Model file for the job. Use its own axes, mm. Round coordinates to 2 decimals unless told otherwise and drop trailing zeros. Loops run counter-clockwise (first coordinate to the right, second up) from the corner with the lowest first, then second, coordinate; pieces in that order, holes last. Notation, with made-up numbers: (-29.5, -10.75) -> (-1.5, -10.75) arc R9 cw to (-1.5, 5.25) -> close; hole circle Ø3 at (88.5, 75). An arc over 180 degrees is marked (long way). Use a Markdown table: item, result.
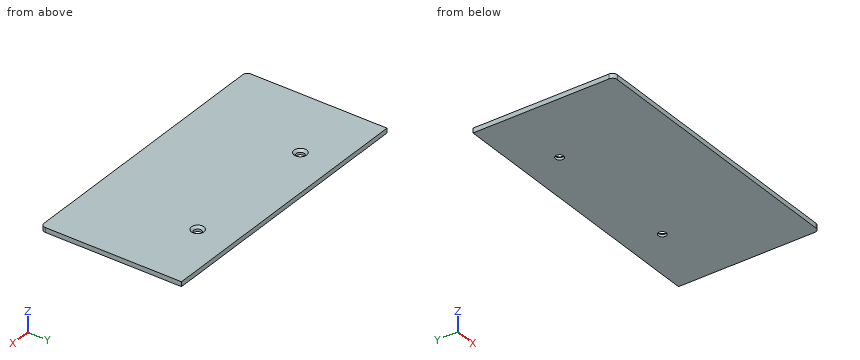
from build123d import *

# Parameters (mm, degrees)
SCHIZZO1_W                   = 120
SCHIZZO1_H                   = 60
SCHIZZO1_R                   = 1.7
ESTRUSIONE_ESTRUSIONE2_DEPTH = 2
RACCORDO1_R                  = 2
RACCORDO2_R                  = 2
SMUSSO1_SIZE                 = 1
SMUSSO2_SIZE                 = 1


with BuildPart() as part:
    # Schizzo1 → Estrusione-Estrusione2 (new body)
    with BuildSketch(Plane.XY):
        with Locations((60, 30)):
            Rectangle(SCHIZZO1_W, SCHIZZO1_H)
        with Locations((90, 45)):
            Circle(SCHIZZO1_R, mode=Mode.SUBTRACT)
        with Locations(Location((30, 45, 0), (0, 0, 180))):
            Circle(SCHIZZO1_R, mode=Mode.SUBTRACT)
    extrude(amount=-ESTRUSIONE_ESTRUSIONE2_DEPTH)

    # Raccordo1
    raccordo1_edges = [part.edges().sort_by_distance(p)[0] for p in [
        (0, 0, -1),
    ]]
    fillet(raccordo1_edges, radius=RACCORDO1_R)

    # Raccordo2
    raccordo2_edges = [part.edges().sort_by_distance(p)[0] for p in [
        (120, 0, -1),
    ]]
    fillet(raccordo2_edges, radius=RACCORDO2_R)

    # Smusso1
    smusso1_edges = [part.edges().sort_by_distance(p)[0] for p in [
        (31.7, 45, 0),
    ]]
    chamfer(smusso1_edges, length=SMUSSO1_SIZE)

    # Smusso2
    smusso2_edges = [part.edges().sort_by_distance(p)[0] for p in [
        (88.3, 45, 0),
    ]]
    chamfer(smusso2_edges, length=SMUSSO2_SIZE)


solid = part.part
Q1. Drill centre lines: L1, parallel to Y at x = 30, z = -1.75; L2, parallel to Y at x = 29, z = -0.4. Where is each one in solid material? Low to high. Write a range as from..to.
Results list:
| item | result |
|---|---|
| L1 | y = 0..43.3, 46.7..60 |
| L2 | y = 0..42.93, 47.07..60 |
Q2. Band-saw the part on A-A, the plane x = 30. Give the cut face in (y, z).
Results list:
| item | result |
|---|---|
| outline | (0, -2) -> (43.3, -2) -> (43.3, -1) -> (42.3, 0) -> (0, 0) -> close; (46.7, -2) -> (60, -2) -> (60, 0) -> (47.7, 0) -> (46.7, -1) -> close |
Q3. Band-saw the part on B-B, the plane y = 45. Give the cut face in (x, z), plus the area to 3 significant figures.
Results list:
| item | result |
|---|---|
| outline | (0, -2) -> (28.3, -2) -> (28.3, -1) -> (27.3, 0) -> (0, 0) -> close; (31.7, -2) -> (88.3, -2) -> (88.3, -1) -> (87.3, 0) -> (32.7, 0) -> (31.7, -1) -> close; (91.7, -2) -> (120, -2) -> (120, 0) -> (92.7, 0) -> (91.7, -1) -> close |
| area | 224 mm² |
